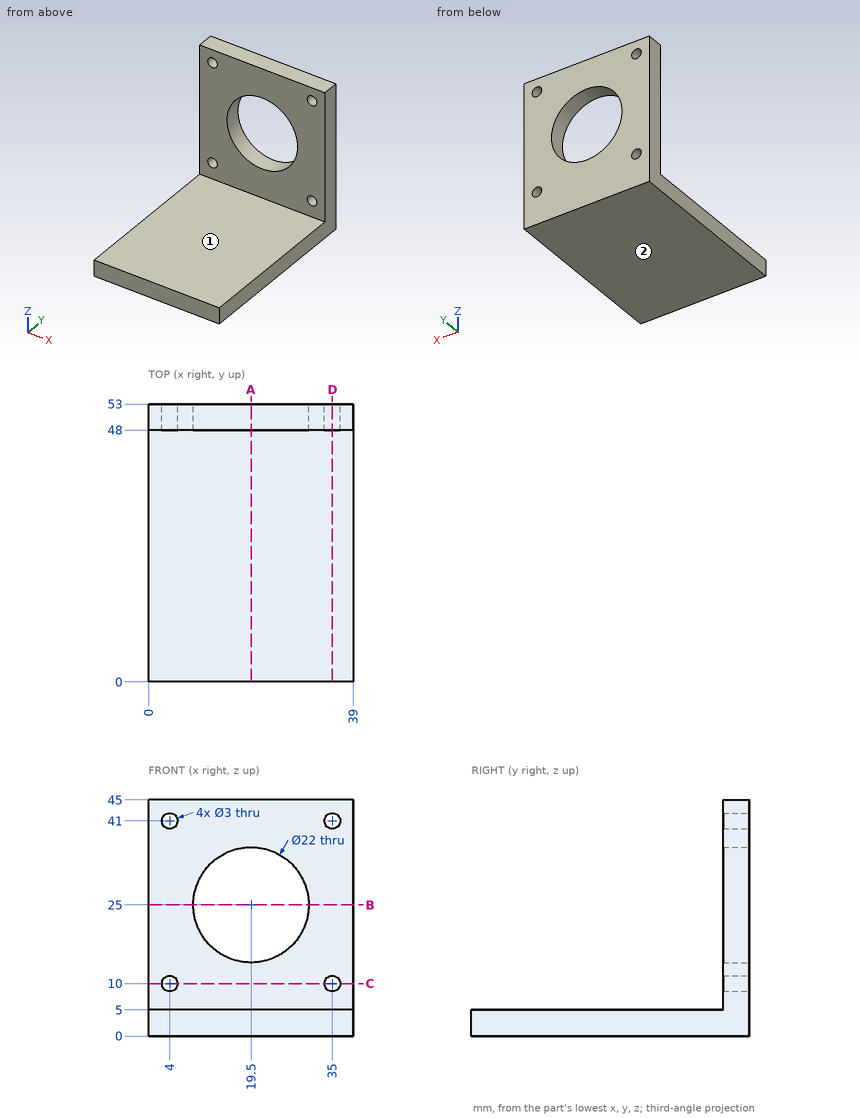
Print and shaded views of the part. All mm, measured from the part's lowest x, y and z. A direction names the side the tool comes from. Coordinates: 2 decimals unless noted, no trailing zeros. Order: outer loops, then holes, each group sorted by start corner. A loop starts at its lowest first (then second) coordinate and runs counter-clockwise, first axis right, second up. Notation, with made-up numbers: (-21.5, 56) - (-13.5, 56) arc R29 cw to (-13.5, 87) - close; hole circle Ø8 at (44, 74.25). An arc over 180 degrees is marked (long way). Put each result on its own line as item: value.
1. Probe line 1 along X through (y, z) = (51, 10); line 2 along Z through (x, y) = (4, 50); line 3 along Z through (x, y) = (35.5, 6). List the from-to ranges inside material, lowest first. Write a range as [from, to].
Answer sheet:
line 1: x = [0, 2.5], [5.5, 33.5], [36.5, 39]
line 2: z = [0, 8.5], [11.5, 39.5], [42.5, 45]
line 3: z = [0, 5]
2. Saw through at C-C (z = 10). Write the cut outline in (x, y), and give its area (3 significant figures).
Answer sheet:
outline: (0, 48) - (2.5, 48) - (2.5, 53) - (0, 53) - close; (5.5, 48) - (33.5, 48) - (33.5, 53) - (5.5, 53) - close; (36.5, 48) - (39, 48) - (39, 53) - (36.5, 53) - close
area: 165 mm^2
3. Saw through at D-D (x = 35). Write the cut outline in (y, z).
Answer sheet:
outline: (0, 0) - (53, 0) - (53, 8.5) - (48, 8.5) - (48, 5) - (0, 5) - close; (48, 11.5) - (53, 11.5) - (53, 39.5) - (48, 39.5) - close; (48, 42.5) - (53, 42.5) - (53, 45) - (48, 45) - close
4. Drop flat-ended pins along their axis: P1, Ø4, axis at x = 28, y = 16.5, coming from the +Z side; P2, Ø12, axis at y = 6, z = 13, coming from the -X side; P3, Ø3.5, axis at x = 35, z = 10, coming from the -Y side. Give the stop position or say it passes through.
Answer sheet:
P1: stops at z = 5
P2: passes through
P3: stops at y = 48
5. Saw through at B-B (z = 25). Write the cut outline in (x, y).
Answer sheet:
outline: (0, 48) - (8.5, 48) - (8.5, 53) - (0, 53) - close; (30.5, 48) - (39, 48) - (39, 53) - (30.5, 53) - close
6. Tool access for the marked faces 1 and 2: list every direction of +Z, -Z, +X, -X, +Y, -Y with a clear straight run to the whole face (end or side of a thin tool).
Answer sheet:
face 1: +Z, +X, -X, -Y
face 2: -Z, +X, -X, +Y, -Y
7. Saw through at A-A (x = 19.5). Write the cut outline in (y, z), and give its area (3 significant figures).
Answer sheet:
outline: (0, 0) - (53, 0) - (53, 14) - (48, 14) - (48, 5) - (0, 5) - close; (48, 36) - (53, 36) - (53, 45) - (48, 45) - close
area: 355 mm^2
